Input: part model. Units: mm. Frame: model coordinates. A direction names the side the tool comes from. Give positions to 0.01 mm unless a question says otherwise; leave off trailing zeros. Loops run counter-clockwise (first coordinate to the right, second up) from the corner with the lowest first, then second, coordinate; pieces in that order, holes last. Notation, with made-up numbers: (5, 46.25) - (58, 46.25) arc R21 cw to (58, 68.25) - close; hole circle Ø1 at (73, -7.5). An arc over 180 degrees is marked (long way). One line per item, written item: value.
from build123d import *

# Parameters (mm, degrees)
SKETCH1_W           = 4
SKETCH1_H           = 16.5
SKETCH1_W_2         = 9
SKETCH1_H_2         = 4
BOSS_EXTRUDE1_DEPTH = 4
FILLET1_R           = 1
SKETCH2_RX          = 13.5
SKETCH2_RY          = 4.5
CUT_EXTRUDE1_DEPTH  = 59.164099752


with BuildPart() as part:
    # Sketch1 → Boss-Extrude1 (new body)
    with BuildSketch(Plane(origin=(0, 0, 0), x_dir=(1, 0, 0), z_dir=(0, 1, 0))):
        Polygon((-18.75, 45), (-18.75, 10), (-23.75, 10), (-23.75, -10), (-18.75, -10), (-18.75, -45), (25.75, -45), (25.75, -22.5), (18.75, -22.5), (18.75, 22.5), (25.75, 22.5), (25.75, 45), (7.5, 45), (7.5, 52), (-7.5, 52), (-7.5, 45), align=None)
        with Locations((20.75, 33.75)):
            Rectangle(SKETCH1_W, SKETCH1_H, mode=Mode.SUBTRACT)
        with Locations((20.75, -33.75)):
            Rectangle(SKETCH1_W, SKETCH1_H, mode=Mode.SUBTRACT)
        with Locations((0, 47)):
            Rectangle(SKETCH1_W_2, SKETCH1_H_2, mode=Mode.SUBTRACT)
        Polygon((-14.75, 7), (-14.75, 36.356853762), (14.75, 7), align=None, mode=Mode.SUBTRACT)
        Polygon((14.75, 12.643146238), (-14.75, 42), (14.75, 42), align=None, mode=Mode.SUBTRACT)
        Polygon((14.75, -7), (-14.75, -36.356853762), (-14.75, -7), align=None, mode=Mode.SUBTRACT)
        Polygon((14.75, -12.643146238), (14.75, -42), (-14.75, -42), align=None, mode=Mode.SUBTRACT)
    extrude(amount=BOSS_EXTRUDE1_DEPTH)

    # Fillet1
    fillet1_edges = [part.edges().sort_by_distance(p)[0] for p in [
        (-14.75, 2, 42),
        (14.75, 2, 42),
        (14.75, 2, 12.643146238),
        (-14.75, 2, 36.356853762),
        (14.75, 2, 7),
        (-14.75, 2, 7),
        (14.75, 2, -42),
        (-14.75, 2, -42),
        (14.75, 2, -12.643146238),
        (14.75, 2, -7),
        (-14.75, 2, -36.356853762),
        (-14.75, 2, -7),
    ]]
    fillet(fillet1_edges, radius=FILLET1_R)

    # Sketch2 → Cut-Extrude1 (cut, through all)
    with BuildSketch(Plane(origin=(0, 4, 0), x_dir=(1, 0, 0), z_dir=(0, 1, 0))):
        with Locations((0, 0)):
            Ellipse(SKETCH2_RX, SKETCH2_RY)
    extrude(amount=-CUT_EXTRUDE1_DEPTH, mode=Mode.SUBTRACT)


solid = part.part
Item 1: Draft query along X for faces 1 (the face through (3, 2, 45)), 2 (the face through (-18.75, 2, 27)), 3 (the face through (22.75, 2, 34)). Return one class per face: pulls with the +X half, pulls with the -X half, needs draft (parallel to the pull), parting line crosses it, or undercut.
Verdict:
face 1: needs draft
face 2: pulls with the -X half
face 3: undercut
Item 2: Section B-B, the plane z = -12.5. Output: boundary loops of the cut face in (x, y), and give its area (3 significant figures).
Verdict:
outline: (-18.75, 0) - (-14.75, 0) - (-14.75, 4) - (-18.75, 4) - close; (9.22, 0) - (18.75, 0) - (18.75, 4) - (9.22, 4) - close
area: 54.1 mm^2
Item 3: Section A-A, the plane z = -36. Output: boundary loops of the cut face in (x, y), and give its area (3 significant figures).
Verdict:
outline: (-18.75, 0) - (-8.72, 0) - (-8.72, 4) - (-18.75, 4) - close; (14.75, 0) - (18.75, 0) - (18.75, 4) - (14.75, 4) - close; (22.75, 0) - (25.75, 0) - (25.75, 4) - (22.75, 4) - close
area: 68.1 mm^2
Item 4: Pin query (flat end, axial travel): P1, Ø1.2, axis at x = -15.5, y = 2.5, coming from the -Z side; P2, Ø1.2, axis at y = 2.5, z = 22.5, coming from the -X side; P3, Ø2, axis at x = -12, z = 24.5, coming from the +Y side. Return the tip coordinate at first contact, or that it passes through.
Verdict:
P1: stops at z = -45
P2: stops at x = -18.75
P3: passes through
Item 5: Section D-D, the plane x = -9.5. Count the separate pieces of the cut face and the enclosed holes in it, and give its area (3 significant figures).
Verdict:
separate pieces: 6
enclosed holes: 0
area: 99.6 mm^2
Item 6: Access query for faces 4 (the face through (-21, 2, 10)), 5 (the face through (21, 2, -25.5)), 6 (the face through (-21, 2, -10)), 7 (the face through (18.75, 2, 0)). Directions: +Z, -Z, +X, -X, +Y, -Y. A direction counts if a zero-diameter tool reaches every point of the face in a straight line with its end or side. Return the directions, or none.
Verdict:
face 4: +Z, -X, +Y, -Y
face 5: +Y, -Y
face 6: -Z, -X, +Y, -Y
face 7: +X, +Y, -Y
Item 7: Section C-C, the plane z = 31. Output: boundary loops of the cut face in (x, y), and give its area (3 significant figures).
Verdict:
outline: (-18.75, 0) - (-14.75, 0) - (-14.75, 4) - (-18.75, 4) - close; (-9.37, 0) - (-3.7, 0) - (-3.7, 4) - (-9.37, 4) - close; (14.75, 0) - (18.75, 0) - (18.75, 4) - (14.75, 4) - close; (22.75, 0) - (25.75, 0) - (25.75, 4) - (22.75, 4) - close
area: 66.7 mm^2
Item 8: Material intervals for L1, parallel to Z at x = 19.5, y = 2.05; L2, parallel to Z at x = 23, y = 2.5; L3, parallel to Z at x = 9, y = 1.3, sorted ascending.
Verdict:
L1: z = -45 to -42, -25.5 to -22.5, 22.5 to 25.5, 42 to 45
L2: z = -45 to -22.5, 22.5 to 45
L3: z = -45 to -42, -18.37 to -12.72, -7 to -3.35, 3.35 to 7, 12.72 to 18.37, 42 to 45
